Study the drawing (mm; zero at the part's minimum x, y, z) and answer. A direction names the side the tool comes from. Round coordinates to 2 decimals unless told otherwise and drop trailing zeros. Write each loop counter-clockwise with the first axis right and the second up, starting at its lowest first coordinate (ties: lowest second). Pieces come first, ordered by that corner, then holes. Notation, with made-up numbers: (-13.75, 64) - (41.25, 64) arc R13 ccw to (41.25, 85) - close; hole circle Ø9 at (-26.5, 11). An arc over 180 degrees is marked (long way). Return JSON: item names as keys, results as strings. Group by question number.
(1) Which of the six approach directions +Z, -Z, +X, -X, +Y, -Y give full straight-line access (tool end or side, diameter ignored) to the marked faces 4, 5, 6 and 7?
(2) Section A-A, the plane y = 101.5 is taken. Write down the section's boundary in (x, z), then the cut area to 3 significant figures.
(3) Each of these flat-tipped pins is pushed along its axis until it touches: pin 1 (6 mm diameter, centred on x = 78.5, z = 27, fed in from +Y); pin 2 (25 mm diameter, centred on x = 30, y = 76, fed in from -Z); pin 3 (15 mm diameter, centred on x = 328.5, z = 133, fed in from +Y). Where does it stop, or does it pass through?
(4) Determine the mould class of the marked faces 1, 2 and 3 for opening direction X: +X half, -X half, draft (parallel to the pull), parting line (faces both ways), or undercut.
(5) Section D-D, the plane y = 50 is taken. Give the number of separate pieces and of enclosed holes in the cut face, then the cut area to 3 significant figures.
(6) Section B-B, the plane x = 316 is taken. Write down the section's boundary in (y, z), then the cut area to 3 significant figures.
(7) Find the intervals of material crossed by line 1 along X through (y, z) = (25.5, 35); line 2 along X through (y, z) = (97, 43); line 3 along Z through (x, y) = (244, 54.5), in increasing order. Write a range as [from, to].
(8) Section C-C, the plane z = 19.5 is taken. Write down the section's boundary in (x, y).
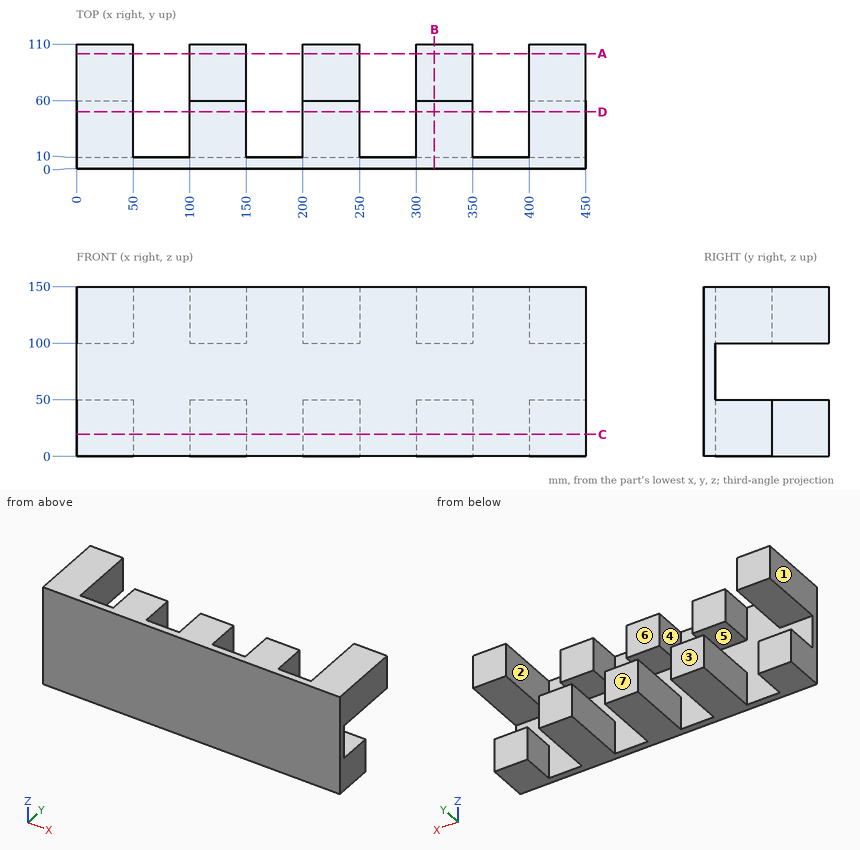
Working result:
{
 "1": {"face 4": "+Z, -Z, +Y", "face 5": "+X, -X, +Y", "face 6": "+Z, +Y", "face 7": "+Z, -Z, +X, -X, +Y"},
 "2": {"outline": "(0, 100) - (50, 100) - (50, 150) - (0, 150) - close; (100, 0) - (150, 0) - (150, 50) - (100, 50) - close; (200, 0) - (250, 0) - (250, 50) - (200, 50) - close; (300, 0) - (350, 0) - (350, 50) - (300, 50) - close; (400, 100) - (450, 100) - (450, 150) - (400, 150) - close", "area": "12,500 mm^2"},
 "3": {"pin 1": "stops at y = 10", "pin 2": "stops at z = 100", "pin 3": "stops at y = 60"},
 "4": {"face 1": "-X half", "face 2": "undercut", "face 3": "draft"},
 "5": {"separate pieces": "10", "enclosed holes": "0", "area": "25,000 mm^2"},
 "6": {"outline": "(0, 0) - (110, 0) - (110, 50) - (10, 50) - (10, 100) - (60, 100) - (60, 150) - (0, 150) - close", "area": "9,000 mm^2"},
 "7": {"line 1": "x = [0, 50], [100, 150], [200, 250], [300, 350], [400, 450]", "line 2": "x = [100, 150], [200, 250], [300, 350]", "line 3": "z = [0, 50], [100, 150]"},
 "8": {"outline": "(0, 0) - (450, 0) - (450, 60) - (400, 60) - (400, 10) - (350, 10) - (350, 110) - (300, 110) - (300, 10) - (250, 10) - (250, 110) - (200, 110) - (200, 10) - (150, 10) - (150, 110) - (100, 110) - (100, 10) - (50, 10) - (50, 60) - (0, 60) - close"}
}
